```python
from build123d import *

# Parameters (mm, degrees)
BASIS_BLECH1_DEPTH             = 1
KANTE_LASCHE2_STRIP_W          = 5.4732
KANTE_LASCHE2_STRIP_H          = 1
KANTE_LASCHE2_STRIP_CUT_DEPTH  = 31.657436361
KANTE_LASCHE2_RELIEF_W         = 5.9732
KANTE_LASCHE2_RELIEF_H         = 0.5
KANTE_LASCHE2_RELIEF_CUT_DEPTH = 1
KANTE_LASCHE2_DEPTH            = 31.657436361
KANTE_LASCHE3_STRIP_CUT_DEPTH  = 11.2634
KANTE_LASCHE3_DEPTH            = 11.2634
VERRUNDUNG1_R                  = 0.5


# Sheet-metal steps are written as plain solids
with BuildPart() as part:
    # Skizze1 → Basis-Blech1 (new body)
    with BuildSketch(Plane.XY):
        with BuildLine():
            Line((-28.342563639, 0.5), (-60, 0.5))
            Line((-60, 0.5), (-60, 6.5))
            ThreePointArc((-60, 6.5), (-59.414213562, 7.914213562), (-58, 8.5))
            Line((-58, 8.5), (-42, 8.5))
            Line((-42, 8.5), (-42, 16.5))
            ThreePointArc((-42, 16.5), (-41.414213562, 17.914213562), (-40, 18.5))
            Line((-40, 18.5), (-22, 18.5))
            ThreePointArc((-22, 18.5), (-18.464466094, 17.035533906), (-17, 13.5))
            Line((-17, 13.5), (-17, 2.5))
            Line((-17, 2.5), (-28.342563639, 0.5))
        make_face()
        with BuildLine():
            Line((-29.75, 7.5), (-29.75, 13.5))
            ThreePointArc((-29.75, 13.5), (-32, 15.75), (-34.25, 13.5))
            Line((-34.25, 13.5), (-34.25, 7.5))
            ThreePointArc((-34.25, 7.5), (-32, 5.25), (-29.75, 7.5))
        make_face(mode=Mode.SUBTRACT)
    extrude(amount=BASIS_BLECH1_DEPTH)

    # Kante-Lasche2 strip (across the edge) → Kante-Lasche2 strip cut (cut)
    with BuildSketch(Plane(origin=(-60, 0.5, 1), x_dir=(0, 1, 0), z_dir=(1, 0, 0))):
        with Locations((-1, -0.5)):
            Rectangle(KANTE_LASCHE2_STRIP_W, KANTE_LASCHE2_STRIP_H)
    extrude(amount=KANTE_LASCHE2_STRIP_CUT_DEPTH, mode=Mode.SUBTRACT)

    # Kante-Lasche2 relief (on the sheet) → Kante-Lasche2 relief cut (cut)
    with BuildSketch(Plane(origin=(-60, 2.2366, 1), x_dir=(0, 1, 0), z_dir=(0, 0, 1))):
        with Locations((-2.4866, -31.907436361)):
            Rectangle(KANTE_LASCHE2_RELIEF_W, KANTE_LASCHE2_RELIEF_H)
    extrude(amount=-KANTE_LASCHE2_RELIEF_CUT_DEPTH, mode=Mode.SUBTRACT)

    # Kante-Lasche2 section (across the edge) → Kante-Lasche2 (add)
    with BuildSketch(Plane(origin=(-60, 0.5, 1), x_dir=(0, 1, 0), z_dir=(1, 0, 0))):
        with BuildLine():
            Line((0, 0.7366), (0, 12))
            Line((0, 12), (1, 12))
            Line((1, 12), (1, 0.7366))
            ThreePointArc((1, 0.7366), (1.215745145, 0.215745145), (1.7366, 0))
            Line((1.7366, 0), (1.7366, -1))
            ThreePointArc((1.7366, -1), (0.508638364, -0.491361636), (0, 0.7366))
        make_face()
    extrude(amount=KANTE_LASCHE2_DEPTH)

    # Kante-Lasche3 strip (across the edge) → Kante-Lasche3 strip cut (cut)
    with BuildSketch(Plane(origin=(-28.342563639, 1.5, 13), x_dir=(-0.1736481776669238, 0.9848077530122092, 3.1093246385391698e-15), z_dir=(0, 0, -1))):
        Polygon((-1.92402835, 5.152936518), (-0.973617144, -0.237113276), (0.011190609, -0.063465098), (-0.939220597, 5.326584696), align=None)
    extrude(amount=KANTE_LASCHE3_STRIP_CUT_DEPTH, mode=Mode.SUBTRACT)

    # Kante-Lasche3 section (across the edge) → Kante-Lasche3 (add)
    with BuildSketch(Plane(origin=(-28.342563639, 1.5, 13), x_dir=(-0.1736481776669238, 0.9848077530122092, 3.1093246385391698e-15), z_dir=(0, 0, -1))):
        with BuildLine():
            Line((-1, 0.06444415), (-1, 11.412511336))
            Line((-1, 11.412511336), (0, 11.412511336))
            Line((0, 11.412511336), (0, 0.06444415))
            ThreePointArc((0, 0.06444415), (0.002802985, 0.000245229), (0.011190609, -0.063465098))
            Line((0.011190609, -0.063465098), (-0.973617144, -0.237113276))
            ThreePointArc((-0.973617144, -0.237113276), (-0.993391713, -0.086910513), (-1, 0.06444415))
        make_face()
    extrude(amount=KANTE_LASCHE3_DEPTH)

    # Verrundung1
    verrundung1_edges = [part.edges().sort_by_distance(p)[0] for p in [
        (-17, 2.5, 0.5),
        (-27.842563639, 0.58816349, 0.5),
    ]]
    fillet(verrundung1_edges, radius=VERRUNDUNG1_R)


solid = part.part
```
The listing builds one solid part. Answer for the finished solid, in the listing's coordinates (mm). A direction names the side the tool comes from. Give positions to 0.01 mm unless a question says otherwise; leave off trailing zeros. Loops run counter-clockwise (first coordinate to the right, second up) from the corner with the lowest first, then second, coordinate; pieces in that order, holes last. Notation, with made-up numbers: (24, 79) - (38, 79) arc R17 ccw to (38, 98) - close; hole circle Ø5 at (78, 45.25). An arc over 180 degrees is marked (long way). Answer as CSV lines item,"result". Start each with the question number.
Item 1: Find the intervals of material crossed by line 1 (Z direction, x = -22, y = 2.5); line 2 (Y direction, x = -32.5, z = 2.5); line 3 (Z direction, x = -21, y = 15), in increasing order. Write a range as from..to.
Item 2: A cutting plane is placed at A-A on x = -32. Determine the outline of the cut face in (y, z).
Item 3: The mould has two halves that part along X. Classify faces 6 (the face through (-22.27, 1.57, 0.49)), 7 (the face through (-34.25, 10.5, 0.5)), 8 (the face through (-31.1, 18.5, 0.5)), 9 (the face through (-41.43, 17.9, 0.49)): +X half, -X half, draft (parallel to the pull), parting line (faces both ways), or undercut.
Item 4: Each of these flat-tipped pins is pushed along its axis until it touches: pin 1 (9 mm diameter, centred on x = -29.5, y = 8, fed in from +Z); pin 2 (0.8 mm diameter, centred on x = -52, z = 0.5, fed in from +Y); pin 3 (2 mm diameter, centred on x = -53, z = 5, fed in from +Y). Where does it stop, or does it pass through?
Item 5: A cutting plane is placed at D-D on x = -24. Determine the outline of the cut face in (y, z).
Item 6: A cutting plane is placed at C-C on x = -44. Determine the outline of the cut face in (y, z).
Item 7: For faces 1 (the face through (-29.75, 10.5, 0.5)), 2 (the face through (-28.343, 1.6, 0.9)), 3 (the face through (-42, 12.4, 0.5)), 4 (the face through (-22.61, 2.51, 7.45)), 5 (the face through (-17.015, 2.982, 7.447)), determine the directions among +Z, -Z, +X, -X, +Y, -Y from which every point of the face is accessible in a straight line to the end or side of a thin tool.
Item 8: A cutting plane is placed at B-B on z = 9.25. Determine the outline of the cut face in (x, y).
Found:
1,line 1,"z = 0..1, 1.74..13"
1,line 2,"y = 0.5..1.5"
1,line 3,"z = 0..1"
2,outline,"(0.5, 1.74) arc R1.74 ccw to (2.24, 0) - (5.25, 0) - (5.25, 1) - (2.24, 1) arc R0.74 cw to (1.5, 1.74) - (1.5, 13) - (0.5, 13) - close; (15.75, 0) - (18.5, 0) - (18.5, 1) - (15.75, 1) - close"
3,face 6,"+X half"
3,face 7,"undercut"
3,face 8,"draft"
3,face 9,"-X half"
4,pin 1,"stops at z = 1"
4,pin 2,"stops at y = 8.5"
4,pin 3,"stops at y = 1.5"
5,outline,"(1.25, 1.74) - (2.27, 1.74) - (2.27, 13) - (1.25, 13) - close; (1.27, 0) - (18.5, 0) - (18.5, 1) - (1.27, 1) - close"
6,outline,"(0.5, 1.74) arc R1.74 ccw to (2.24, 0) - (8.5, 0) - (8.5, 1) - (2.24, 1) arc R0.74 cw to (1.5, 1.74) - (1.5, 13) - (0.5, 13) - close"
7,face 1,"+Z, -Z"
7,face 2,"-Z, -Y"
7,face 3,"+Z, -Z, -X, +Y"
7,face 4,"+Z, -X, +Y"
7,face 5,"+Z, +X, +Y"
8,outline,"(-60, 0.5) - (-28.41, 0.5) arc R1.74 ccw to (-28.11, 0.53) - (-16.93, 2.5) - (-17.1, 3.48) - (-28.28, 1.51) arc R0.74 cw to (-28.41, 1.5) - (-60, 1.5) - close"
